Here's how the part is built. I have some questions about the finished solid (model axes, mm). A direction names the side the tool comes from. Coordinates: 2 decimals unless noted, no trailing zeros. Write each loop counter-clockwise with the first axis right and the second up, starting at its lowest first coordinate (ties: lowest second). Pieces come first, ordered by that corner, then holes. Notation, with made-up numbers: (72.5, -23) -> (98.5, -23) arc R11 cw to (98.5, -14) -> close; hole circle Ø11 at (83.5, 23). An arc over 180 degrees is marked (long way). Use a Markdown table: item, result. Add a question column.
Item 1: Imagine slicing it at B-B, the plane z = 3.75. Count the separate pieces of the cut face and the enclosed holes in it, and give its area (3 significant figures).
Item 2: Imagine slicing it at A-A, the plane y = -31.5. Write out the boundary of the cut face in (x, z), and give its area (3 significant figures).
Item 3: Will this pin go through, and if not, where does the flat tip stop? pin 1 Ø1.9 at (x, z) = (90.5, 2) entering from -Y.
Item 4: On a 3-axis mill with a long thin cutter (end or side, diameter ignored), from which of +Z, -Z, +X, -X, +Y, -Y can I reach the whole of each face in a straight line? I mean faces 1 (the flat face through (88.138, -3, 3)), 2 (the flat face through (88.138, -60, 3)), 3 (the flat face through (217, -31, 5.08)). Say none if no direction works.
Item 5: If I drill on line 1 along Y through (x, z) = (171.5, 1.75); line 2 along X through (y, z) = (-3, 3.25); line 3 along X through (y, z) = (-54.5, 4), over which ranges is the centre line in solid material (lowest first)? Write a range as from..to.
```python
from build123d import *

# Parameters (mm, degrees)
SKETCH1_W                       = 257.81
SKETCH1_H                       = 63.5
BOSS_EXTRUDE1_DEPTH             = 6.35
CUT_EXTRUDE2_DEPTH              = 1.27
CUT_EXTRUDE3_DEPTH              = 266.590979892
F_6_CLEARANCE_HOLE1_D           = 3.7973
F_6_CLEARANCE_HOLE1_CSINK_D     = 5.0673
F_6_CLEARANCE_HOLE1_CSINK_ANGLE = 90


with BuildPart() as part:
    # Sketch1 → Boss-Extrude1 (new body)
    with BuildSketch(Plane.XY):
        with Locations((128.905, -31.75)):
            Rectangle(SKETCH1_W, SKETCH1_H)
    extrude(amount=BOSS_EXTRUDE1_DEPTH)

    # Sketch4 → Cut-Extrude2 (cut)
    with BuildSketch(Plane.XY.offset(6.35)):
        Polygon((128.905, -20.32), (125.147923653, -28.377076227), (116.257923653, -28.377076227), (123.068058752, -34.091458077), (120.767157441, -42.678538673), (128.905, -39.09976535), (137.042842559, -42.678538673), (134.741941248, -34.091458077), (141.552076347, -28.377076227), (132.662076347, -28.377076227), align=None)
        Polygon((217.17, -20.32), (213.412923653, -28.377076227), (204.522923653, -28.377076227), (211.333058752, -34.091458077), (209.032157441, -42.678538673), (217.17, -39.09976535), (225.307842559, -42.678538673), (223.006941248, -34.091458077), (229.817076347, -28.377076227), (220.927076347, -28.377076227), align=None)
        Polygon((40.64, -20.32), (36.882923653, -28.377076227), (27.992923653, -28.377076227), (34.803058752, -34.091458077), (32.502157441, -42.678538673), (40.64, -39.09976535), (48.777842559, -42.678538673), (46.476941248, -34.091458077), (53.287076347, -28.377076227), (44.397076347, -28.377076227), align=None)
    extrude(amount=-CUT_EXTRUDE2_DEPTH, mode=Mode.SUBTRACT)

    # Sketch6 → Cut-Extrude3 (cut, through all)
    with BuildSketch(Plane.XY.offset(6.35)):
        Polygon((88.138, 0), (91.948, 0), (91.948, -6.35), (94.488, -6.35), (94.488, -10.16), (91.948, -10.16), (91.948, -12.7), (88.138, -12.7), (88.138, -10.16), (85.598, -10.16), (85.598, -6.35), (88.138, -6.35), align=None)
        Polygon((165.862, 0), (169.672, 0), (169.672, -6.35), (172.212, -6.35), (172.212, -10.16), (169.672, -10.16), (169.672, -12.7), (165.862, -12.7), (165.862, -10.16), (163.322, -10.16), (163.322, -6.35), (165.862, -6.35), align=None)
        Polygon((88.138, -63.5), (91.948, -63.5), (91.948, -57.15), (94.488, -57.15), (94.488, -53.34), (91.948, -53.34), (91.948, -50.8), (88.138, -50.8), (88.138, -53.34), (85.598, -53.34), (85.598, -57.15), (88.138, -57.15), align=None)
        Polygon((165.862, -63.5), (169.672, -63.5), (169.672, -57.15), (172.212, -57.15), (172.212, -53.34), (169.672, -53.34), (169.672, -50.8), (165.862, -50.8), (165.862, -53.34), (163.322, -53.34), (163.322, -57.15), (165.862, -57.15), align=None)
    extrude(amount=-CUT_EXTRUDE3_DEPTH, mode=Mode.SUBTRACT)

    # #6 Clearance Hole1 (through all)
    with Locations(Plane.XY.offset(6.35)):
        with Locations((3.175, -16.764), (3.175, -46.736), (254.635, -46.736), (254.635, -16.764)):
            CounterSinkHole(F_6_CLEARANCE_HOLE1_D / 2, F_6_CLEARANCE_HOLE1_CSINK_D / 2, counter_sink_angle=F_6_CLEARANCE_HOLE1_CSINK_ANGLE)


solid = part.part
```
Ans:
| question | item | result |
|---|---|---|
| 1 | separate pieces | 1 |
| 1 | enclosed holes | 4 |
| 1 | area | 16,100 mm^2 |
| 2 | outline | (0, 0) -> (257.81, 0) -> (257.81, 6.35) -> (226.1, 6.35) -> (226.1, 5.08) -> (208.24, 5.08) -> (208.24, 6.35) -> (137.83, 6.35) -> (137.83, 5.08) -> (119.98, 5.08) -> (119.98, 6.35) -> (49.57, 6.35) -> (49.57, 5.08) -> (31.71, 5.08) -> (31.71, 6.35) -> (0, 6.35) -> close |
| 2 | area | 1,570 mm^2 |
| 3 | pin 1 | stops at y = -50.8 |
| 4 | face 1 | +Z, -Z, +Y |
| 4 | face 2 | +Z, -Z, -Y |
| 4 | face 3 | +Z |
| 5 | line 1 | y = -63.5..-57.15, -53.34..-10.16, -6.35..0 |
| 5 | line 2 | x = 0..88.14, 91.95..165.86, 169.67..257.81 |
| 5 | line 3 | x = 0..85.6, 94.49..163.32, 172.21..257.81 |
